Work out the finished part from the listing and answer in its coordinate system (mm). Face numbers are marked on the shaded views. A direction names the side the tool comes from. Round coordinates to 2 decimals unless told otherwise and drop trailing zeros. Loops run counter-clockwise (first coordinate to the right, second up) from the corner with the lowest first, then second, coordinate; pieces in that order, holes last.
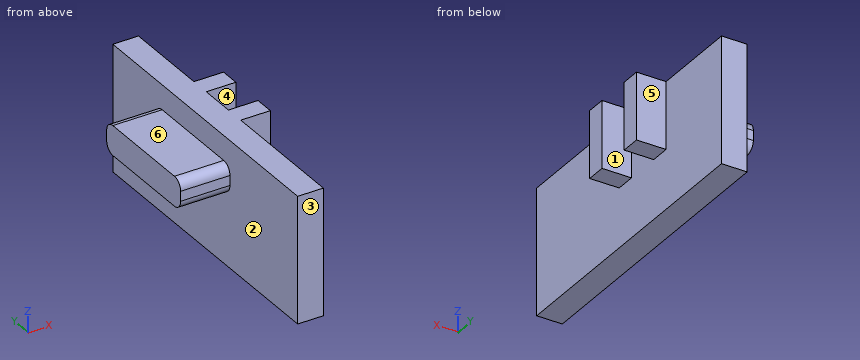
```python
from build123d import *

# Parameters (mm, degrees)
SKETCH019_W  = 15
SKETCH019_H  = 6.4
PAD010_DEPTH = 1.3
SKETCH020_W  = 6
SKETCH020_H  = 1.5
PAD011_DEPTH = 2.5
SKETCH021_W  = 1
SKETCH021_H  = 3.4
PAD012_DEPTH = 1.5
FILLET_R     = 0.5


with BuildPart() as part:
    # Sketch019 → Pad010 (new body)
    with BuildSketch(Plane.YZ.offset(3.6)):
        with Locations((78.3, 5.2)):
            Rectangle(SKETCH019_W, SKETCH019_H)
    extrude(amount=-PAD010_DEPTH)

    # Sketch020 (on Face6 of Pad010) → Pad011 (join)
    with BuildSketch(Plane(origin=(2.3, 0, 0), x_dir=(0, 1, 0), z_dir=(-1, 0, 0))):
        with Locations((79.3, -6.4)):
            Rectangle(SKETCH020_W, SKETCH020_H)
    extrude(amount=PAD011_DEPTH)

    # Sketch021 (on Face4 of Pad011) → Pad012 (join)
    with BuildSketch(Plane.YZ.offset(3.6)):
        with Locations((78, 6.7)):
            Rectangle(SKETCH021_W, SKETCH021_H)
        with Locations((80.8, 6.7)):
            Rectangle(SKETCH021_W, SKETCH021_H)
    extrude(amount=PAD012_DEPTH)

    # Fillet
    fillet_edges = [part.edges().sort_by_distance(p)[0] for p in [
        (1.05, 76.3, 7.15),
        (1.05, 76.3, 5.65),
        (1.05, 82.3, 5.65),
        (1.05, 82.3, 7.15),
    ]]
    fillet(fillet_edges, radius=FILLET_R)


solid = part.part
```
1. Which of the six approach directions +Z, -Z, +X, -X, +Y, -Y give full straight-line access (tool end or side, diameter ignored) to the marked faces 4, 5 and 6?
Answer key:
face 4: +Z, -Z, +X
face 5: +Z, -Z, +X, +Y
face 6: +Z, -X, +Y, -Y
2. Given pin 1 (1 mm diameter, centred on y = 84, z = 4.5, fed in from -X); pin 2 (1.6 mm diameter, centred on x = 4.5, z = 7, fed in from -Y); pin 3 (1.2 mm diameter, centred on x = 1, y = 79, fed in from +Z), each flat-ended and moving along its own axis, determine where each tip first touches the part or whether it passes through.
Answer key:
pin 1: stops at x = 2.3
pin 2: stops at y = 77.5
pin 3: stops at z = 7.15
3. Find section B-B (x = 0.6). Write down the section's boundary in (y, z), then the cut area to 3 significant figures.
Answer key:
outline: (76.3, 6.15) arc R0.5 ccw to (76.8, 5.65) - (81.8, 5.65) arc R0.5 ccw to (82.3, 6.15) - (82.3, 6.65) arc R0.5 ccw to (81.8, 7.15) - (76.8, 7.15) arc R0.5 ccw to (76.3, 6.65) - close
area: 8.79 mm2
4. Determine the mould class of the marked faces 1, 2 and 3 for opening direction Y: +Y half, -Y half, draft (parallel to the pull), parting line (faces both ways), or undercut.
Answer key:
face 1: undercut
face 2: draft
face 3: -Y half
5. Find section C-C (y = 79.5). Write down the section's boundary in (x, z), then the cut area to 3 significant figures.
Answer key:
outline: (-0.2, 5.65) - (2.3, 5.65) - (2.3, 2) - (3.6, 2) - (3.6, 8.4) - (2.3, 8.4) - (2.3, 7.15) - (-0.2, 7.15) - close
area: 12.1 mm2
6. Consider probe 1 along X at (y, z) = (76.25, 6.25); probe 2 along Y at (x, z) = (0.5, 6.5); probe 3 along Y at (x, z) = (2.05, 7). Determine where each line is inside the solid, lowest interval first.
Answer key:
probe 1: x = 2.3 to 3.6
probe 2: y = 76.3 to 82.3
probe 3: y = 76.44 to 82.16
7. Find section D-D (z = 6.5). Write down the section's boundary in (x, y), then the cut area to 3 significant figures.
Answer key:
outline: (-0.2, 76.3) - (2.3, 76.3) - (2.3, 70.8) - (3.6, 70.8) - (3.6, 77.5) - (5.1, 77.5) - (5.1, 78.5) - (3.6, 78.5) - (3.6, 80.3) - (5.1, 80.3) - (5.1, 81.3) - (3.6, 81.3) - (3.6, 85.8) - (2.3, 85.8) - (2.3, 82.3) - (-0.2, 82.3) - close
area: 37.5 mm2
8. Find section A-A (z = 7.5). Write down the section's boundary in (x, y), then the cut area to 3 significant figures.
Answer key:
outline: (2.3, 70.8) - (3.6, 70.8) - (3.6, 77.5) - (5.1, 77.5) - (5.1, 78.5) - (3.6, 78.5) - (3.6, 80.3) - (5.1, 80.3) - (5.1, 81.3) - (3.6, 81.3) - (3.6, 85.8) - (2.3, 85.8) - close
area: 22.5 mm2
